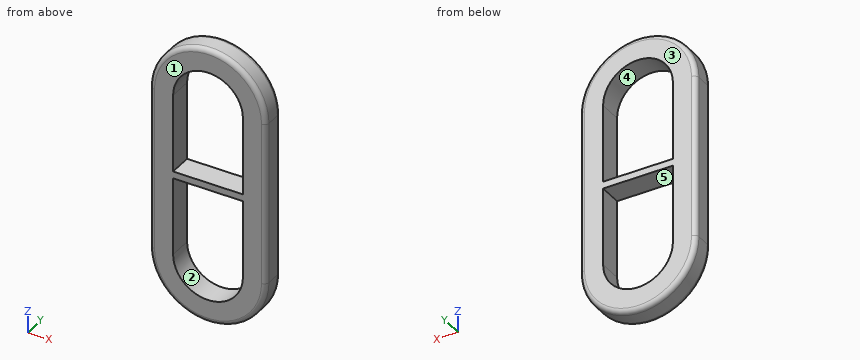
Autodesk Inventor part; units mm, degrees
ref_plane "YZ Plane" through (0, 0, 0) normal (1, 0, 0) x (0, 1, 0)
ref_plane "XZ Plane" through (0, 0, 0) normal (0, 1, 0) x (-1, 0, 0)
ref_plane "XY Plane" through (0, 0, 0) normal (0, 0, 1) x (1, 0, 0)
sketch "Boceto1" plane through (0, 0, 0) normal (0, 1, 0) x (-1, 0, 0)
  line L0 (0, 35) -> (0, -35) construction
  line L1 (25, 35) -> (25, -35)
  line L2 (-25, -35) -> (-25, 35)
  arc A0 (25, 35) -> (-25, 35) centre (0, 35) ccw
  arc A1 (-25, -35) -> (25, -35) centre (0, -35) ccw
  circle A2 centre (0, -35) radius 15
  circle A3 centre (0, 35) radius 15
  line L3 (0, -20) -> (0, -20)
  line L4 (15, -35) -> (-15, -35)
  line L5 (94.5074, 0) -> (-76.0102, 0) construction
  line L6 (15, 35) -> (-15, 35)
  line L7 (15, -35) -> (-15, -35)
  line L8 (-15, -35) -> (-15, -1.5)
  line L9 (-15, -1.5) -> (15, -1.5)
  line L10 (15, -1.5) -> (15, -35)
  line L11 (-15, 35) -> (-15, 1.5)
  line L12 (-15, 1.5) -> (15, 1.5)
  line L13 (15, 1.5) -> (15, 35)
  point P0 (0, 0)
  point P1 (0, 60)
  point P2 (0, -60)
  point P3 (0, -20)
  point P4 (15, 35)
  point P5 (15, 35)
  dimension "largo" = 120
  dimension "d1" = 50
  dimension "espesor_junta" = 10
  dimension "d3" = 10
  dimension "d6" = 0
  dimension "d9" = 1.5
extrude "Extrusión2" add sketch "Boceto1" along normal blind 10
fillet "Empalme1" radius 2 8 edges at (0, 10, 60) (25, 10, 0) (0, 10, -60) (-25, 10, 0) (0, 0, -60) (-25, 0, 0) (0, 0, 60) (25, 0, 0)
equation "\"d3\" = espesor_junta"
properties part number "mod2" material "Aluminio 6061"
Read the model definition and answer for the solid it produces. Units are mm, in the model's axes. Face numbers are marked on the shaded views. A direction names the side the tool comes from. Coordinates: 2 decimals unless noted, no trailing zeros. Write each loop counter-clockwise with the first axis right and the second up, starting at its lowest first coordinate (ties: lowest second). Pieces come first, ordered by that corner, then holes. Notation, with made-up numbers: M -29,85 L -1,85 A9 ccw -1,101 Z; hole C -10.75,77 d4. An arc over 180 degrees is marked long. Use a Markdown table: item, result.
Q1. Straight lines are drawn through the part: L1, parallel to Z at x = -1, y = 9.25; L2, parallel to Z at x = -13, y = 4.75; L3, parallel to X at y = 1.75, z = 21. For each, find the intervals that lie inside material, in ascending order. Write a range as [from, to].
Answer block:
| item | result |
|---|---|
| L1 | z = [-59.54, -49.97], [-1.5, 1.5], [49.97, 59.54] |
| L2 | z = [-56.35, -42.48], [-1.5, 1.5], [42.48, 56.35] |
| L3 | x = [-24.98, -15], [15, 24.98] |
Q2. The part is cut by section A-A, the plane z = -27.5. Write down the section's boundary in (x, y).
Answer block:
| item | result |
|---|---|
| outline | M -25,2 A2 ccw -23,0 L -15,0 L -15,10 L -23,10 A2 ccw -25,8 Z; M 15,0 L 23,0 A2 ccw 25,2 L 25,8 A2 ccw 23,10 L 15,10 Z |
Q3. Which of the six approach directions +Z, -Z, +X, -X, +Y, -Y give full straight-line access (tool end or side, diameter ignored) to the marked faces 1 and 2?
Answer block:
| item | result |
|---|---|
| face 1 | +Z, -Z, +X, -X, -Y |
| face 2 | +Y, -Y |
Q4. The part is cut by section B-B, the plane x = 0. Write down the section's boundary in (y, z).
Answer block:
| item | result |
|---|---|
| outline | M 0,-58 A2 ccw 2,-60 L 8,-60 A2 ccw 10,-58 L 10,-50 L 0,-50 Z; M 0,-1.5 L 10,-1.5 L 10,1.5 L 0,1.5 Z; M 0,50 L 10,50 L 10,58 A2 ccw 8,60 L 2,60 A2 ccw 0,58 Z |
Q5. Each of these flat-tipped pins is pushed along its axis until it touches: pin 1 Ø4 at (x, y) = (-4, 2.5) entering from +Z; pin 2 Ø5 at (x, y) = (4.5, 6) entering from -Z; pin 3 Ø1.5 at (x, y) = (-13, 1.5) entering from -Z. Where does it stop, or does it pass through?
Answer block:
| item | result |
|---|---|
| pin 1 | stops at z = 59.92 |
| pin 2 | stops at z = -59.92 |
| pin 3 | stops at z = -56.75 |
Q6. Determine the mould class of the marked faces 3, 4 and 5 for opening direction X: released by +X, released by -X, zero draft, split by the parting line, or undercut.
Answer block:
| item | result |
|---|---|
| face 3 | zero draft |
| face 4 | undercut |
| face 5 | undercut |
Q7. The part is cut by section C-C, the plane x = 7. Give the number of separate pieces and of enclosed holes in the cut face, then the cut area to 3 significant figures.
Answer block:
| item | result |
|---|---|
| separate pieces | 3 |
| enclosed holes | 0 |
| area | 241 mm2 |
